```python
from build123d import *

# Parameters (mm, degrees)
SKETCH1_W             = 40
SKETCH1_H             = 10
BOSS_EXTRUDE1_DEPTH   = 2
FILLET1_R             = 3
F_3_0MM_DOWEL_HOLE1_D = 3


with BuildPart() as part:
    # Sketch1 → Boss-Extrude1 (new body)
    with BuildSketch(Plane(origin=(0, 0, 0), x_dir=(1, 0, 0), z_dir=(0, 1, 0))):
        Rectangle(SKETCH1_W, SKETCH1_H)
    extrude(amount=BOSS_EXTRUDE1_DEPTH)

    # Fillet1
    fillet1_edges = [part.edges().sort_by_distance(p)[0] for p in [
        (20, 1, 5),
        (-20, 1, 5),
        (-20, 1, -5),
        (20, 1, -5),
    ]]
    fillet(fillet1_edges, radius=FILLET1_R)

    # Ø3.0mm Dowel Hole1 (through all)
    with Locations(Plane(origin=(0, 2, 0), x_dir=(1, 0, 0), z_dir=(0, 1, 0))):
        with Locations((16, 0), (-16, 0)):
            Hole(F_3_0MM_DOWEL_HOLE1_D / 2)


solid = part.part
```
Read the model definition and answer for the solid it produces. Units are mm, in the model's axes. Coordinates: 2 decimals unless noted, no trailing zeros. Loops run counter-clockwise (first coordinate to the right, second up) from the corner with the lowest first, then second, coordinate; pieces in that order, holes last.
(1) Flat-ended cylindrical pins translate along their axes: pin 1 Ø5 at (x, z) = (16, 0) entering from -Y; pin 2 Ø1 at (y, z) = (0.5, -3) entering from +X. Find the tip coordinate at first contact, or state that the pin passes through.
Solution:
pin 1: stops at y = 0
pin 2: stops at x = 19.96
(2) The mould has two halves that part along Z. Classify faces 1 (the face through (19.14, 1.01, -4.1)), 2 (the face through (-14.5, 0.99, -0.07)), 3 (the face through (-20, 1, 0)): released by +Z, released by -Z, zero draft, split by the parting line, or undercut.
Solution:
face 1: released by -Z
face 2: undercut
face 3: zero draft
(3) The part is cut by section D-D (z = 4). Determine the outline of the cut face in (x, y).
Solution:
outline: (-19.24, 0) - (19.24, 0) - (19.24, 2) - (-19.24, 2) - close
(4) The part is cut by section B-B (y = 0.6). Determine the outline of the cut face in (x, z).
Solution:
outline: (-20, -2) arc R3 ccw to (-17, -5) - (17, -5) arc R3 ccw to (20, -2) - (20, 2) arc R3 ccw to (17, 5) - (-17, 5) arc R3 ccw to (-20, 2) - close; hole circle Ø3 at (-16, 0); hole circle Ø3 at (16, 0)
(5) Consider line 1 along Z through (x, y) = (-16, 0.75); line 2 along X through (y, z) = (1.15, -1); line 3 along X through (y, z) = (1, 1.25). Determine where each line is inside the solid, lowest interval first.
Solution:
line 1: z = -5 to -1.5, 1.5 to 5
line 2: x = -20 to -17.12, -14.88 to 14.88, 17.12 to 20
line 3: x = -20 to -16.83, -15.17 to 15.17, 16.83 to 20
(6) The part is cut by section C-C (z = 0). Determine the outline of the cut face in (x, y), and give its area (3 significant figures).
Solution:
outline: (-20, 0) - (-17.5, 0) - (-17.5, 2) - (-20, 2) - close; (-14.5, 0) - (14.5, 0) - (14.5, 2) - (-14.5, 2) - close; (17.5, 0) - (20, 0) - (20, 2) - (17.5, 2) - close
area: 68.0 mm2
(7) The part is cut by section A-A (x = -16). Determine the outline of the cut face in (y, z), and give its area (3 significant figures).
Solution:
outline: (0, -5) - (2, -5) - (2, -1.5) - (0, -1.5) - close; (0, 1.5) - (2, 1.5) - (2, 5) - (0, 5) - close
area: 14.0 mm2
